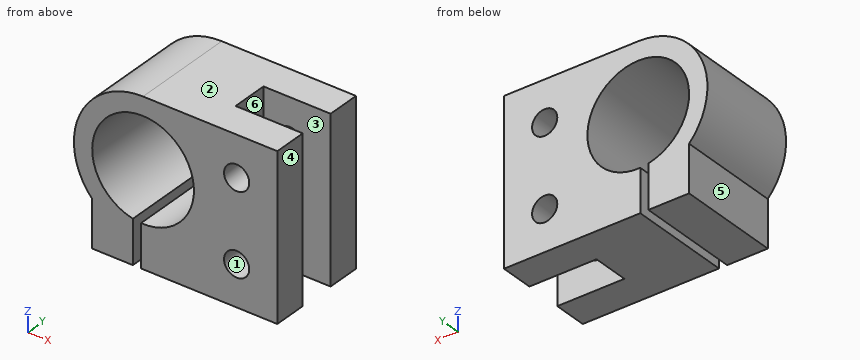
Autodesk Inventor part; units mm, degrees
ref_plane "YZ Plane" through (0, 0, 0) normal (1, 0, 0) x (0, 1, 0)
ref_plane "XZ Plane" through (0, 0, 0) normal (0, 1, 0) x (-1, 0, 0)
ref_plane "XY Plane" through (0, 0, 0) normal (0, 0, 1) x (1, 0, 0)
sketch "Sketch1" plane through (0, 0, 0) normal (0, 1, 0) x (-1, 0, 0)
  line L0 (50, 0) -> (50, 40)
  line L1 (50, 40) -> (0, 40)
  line L2 (0, 40) -> (0, 0)
  line L3 (0, 0) -> (10, 0)
  line L4 (10, 0) -> (10, 10)
  line L5 (10, 10) -> (10, 30)
  circle A0 centre (10, 30) radius 3.1
  circle A1 centre (10, 10) radius 3.1
  line L6 (45.5, 0) -> (45.5, 11.4783)
  line L7 (0, 0) -> (33.5, 0)
  line L8 (35.5, 0) -> (35.5, 10.7526)
  line L9 (50, 40) -> (45.5, 40)
  line L10 (45.5, 40) -> (45.5, 35.5)
  line L11 (45.5, 35.5) -> (45.5, 34.5217)
  line L12 (45.5, 23) -> (33, 23)
  arc A2 (35.5, 10.7526) -> (33.5, 10.51) centre (33, 23) ccw
  arc A3 (45.5, 11.4783) -> (33, 40) centre (33, 23) ccw
  line L13 (0, 0) -> (33.5, 0)
  line L14 (35.5, 0) -> (45.5, 0)
  line L15 (33.5, 0) -> (33.5, 10.51)
  line L16 (0, 0) -> (33.5, 0)
  line L17 (35.5, 0) -> (45.5, 0)
  dimension "d0" = 50
  dimension "d1" = 40
  dimension "d2" = 10
  dimension "d3" = 10
  dimension "d4" = 20
  dimension "d5" = 6.2
  dimension "d6" = 6.2
  dimension "d7" = 45.5
  dimension "d8" = 35.5
  dimension "d9" = 4.5
  dimension "d10" = 4.5
  dimension "d11" = 12.5
  dimension "d12" = 12.5
  dimension "d13" = 2
extrude "Extrusion1" add sketch "Sketch1" along normal blind 25.4 contours A3 L6 L14 L8 A2 L15 L7 L3 L2 L1
sketch "Sketch2" plane through (-33, 0, 40) normal (0, 0, 1) x (1, 0, 0)
  line L0 (33, 0) -> (33, 8.2)
  line L1 (33, 0) -> (33, 25.4)
  line L2 (33, 8.2) -> (16.5, 8.2)
  line L3 (16.5, 8.2) -> (16.5, 17.2)
  line L4 (16.5, 17.2) -> (33, 17.2)
  line L5 (33, 17.2) -> (33, 8.2)
  dimension "d16" = 8.2
  dimension "d17" = 16.5
  dimension "d18" = 9
extrude "Extrusion2" cut sketch "Sketch2" against normal through all
properties part number "suporte-eixo-new" material "Steel, Carbon"
The listing builds one solid part. Answer for the finished solid, in the listing's coordinates (mm). Face numbers are marked on the shaded views. A direction names the side the tool comes from. Give positions to 0.01 mm unless a question says otherwise; leave off trailing zeros. Order: outer loops, then holes, each group sorted by start corner. A loop starts at its lowest first (then second) coordinate and runs counter-clockwise, first axis right, second up. Notation, with made-up numbers: M 31,79.25 L 73,79.25 A14 cw 73,89.25 Z; hole C -6,41.5 d8. An arc over 180 degrees is marked long. Put each result on its own line as item: value. Start each with the question number.
Item 1: The part is cut by section D-D, the plane z = 5. Determine the outline of the cut face in (x, y), and give its area (3 significant figures).
Item 2: The part is cut by section B-B, the plane y = 5.5. Determine the outline of the cut face in (x, z), and give its area (3 significant figures).
Item 3: The part is cut by section C-C, the plane x = -10. Determine the outline of the cut face in (y, z), and give its area (3 significant figures).
Item 4: Which of the six approach directions +Z, -Z, +X, -X, +Y, -Y give full straight-line access (tool end or side, diameter ignored) to the marked faces 4, 5 and 6?
Item 5: Flat-ended cylindrical pins translate along their axes: P1, Ø4, axis at y = 12.5, z = 9, coming from the -X side; P2, Ø5.5, axis at x = -10, z = 30, coming from the -Y side. Find the tip coordinate at first contact, or state that the pin passes through.
Item 6: The part is cut by section A-A, the plane x = -3.5. Determine the outline of the cut face in (y, z), and give its area (3 significant figures).
Item 7: For a pull along Z with two mould halves and no side action, classify the marked faces 1, 2 and 3 as +Z half, -Z half, draft (parallel to the pull), parting line (faces both ways), or undercut.
Item 8: Find the intervals of material crossed by line 1 along Z through (x, y) = (-10, 2.5); line 2 along X through (y, z) = (23.75, 10); line 3 along Y through (x, z) = (-7.5, 34.5), in increasing order.
Answer key:
1. outline: M -45.5,0 L -35.5,0 L -35.5,25.4 L -45.5,25.4 Z; M -33.5,0 L 0,0 L 0,8.2 L -16.5,8.2 L -16.5,17.2 L 0,17.2 L 0,25.4 L -33.5,25.4 Z
1. area: 956 mm²
2. outline: M -45.5,0 L -35.5,0 L -35.5,10.75 A12.5 cw long -33.5,10.51 L -33.5,0 L 0,0 L 0,40 L -33,40 A17 ccw -45.5,11.48 Z; hole C -10,10 d6.2; hole C -10,30 d6.2
2. area: 1,300 mm²
3. outline: M 0,0 L 8.2,0 L 8.2,6.9 L 0,6.9 Z; M 0,13.1 L 8.2,13.1 L 8.2,26.9 L 0,26.9 Z; M 0,33.1 L 8.2,33.1 L 8.2,40 L 0,40 Z; M 17.2,0 L 25.4,0 L 25.4,6.9 L 17.2,6.9 Z; M 17.2,13.1 L 25.4,13.1 L 25.4,26.9 L 17.2,26.9 Z; M 17.2,33.1 L 25.4,33.1 L 25.4,40 L 17.2,40 Z
3. area: 453 mm²
4. face 4: +Z, -Z, +X, +Y, -Y
4. face 5: -Z, -X, +Y, -Y
4. face 6: +Z, -Z, +X
5. P1: stops at x = -45.5
5. P2: passes through
6. outline: M 0,0 L 8.2,0 L 8.2,40 L 0,40 Z; M 17.2,0 L 25.4,0 L 25.4,40 L 17.2,40 Z
6. area: 656 mm²
7. face 1: undercut
7. face 2: +Z half
7. face 3: draft
8. line 1: z = 0 to 6.9, 13.1 to 26.9, 33.1 to 40
8. line 2: x = -45.5 to -35.5, -33.5 to -13.1, -6.9 to 0
8. line 3: y = 0 to 8.2, 17.2 to 25.4
